```python
from build123d import *

# Parameters (mm, degrees)
SKETCH1_W               = 10
SKETCH1_H               = 10
BASE_FLANGE1_DEPTH      = 1
EDGE_FLANGE2_DEPTH      = 10
EDGE_FLANGE2_BEND_DEPTH = 10
EDGE_FLANGE3_DEPTH      = 10
EDGE_FLANGE3_BEND_DEPTH = 10
CUT_EXTRUDE1_DEPTH      = 10
SKETCH25_R              = 2.5
CUT_EXTRUDE2_DEPTH      = 10
SKETCH26_R              = 2.5
CUT_EXTRUDE3_DEPTH      = 10
SKETCH27_R              = 2.5
CUT_EXTRUDE4_DEPTH      = 1


# Sheet-metal steps are written as plain solids
with BuildPart() as part:
    # Sketch1 → Base-Flange1 (new body)
    with BuildSketch(Plane(origin=(0, 0, 0), x_dir=(1, 0, 0), z_dir=(0, 1, 0))):
        with Locations((0, 0.042787107)):
            Rectangle(SKETCH1_W, SKETCH1_H)
    extrude(amount=-BASE_FLANGE1_DEPTH)

    # Edge-Flange2 section (across the edge) → Edge-Flange2 (add)
    with BuildSketch(Plane(origin=(5.7366, -1, -5.042787107), x_dir=(-1, 0, 0), z_dir=(0, 0, 1))):
        with BuildLine():
            Line((-1, 0.7366), (-1, 9))
            Line((-1, 9), (0, 9))
            Line((0, 9), (0, 0.7366))
            ThreePointArc((0, 0.7366), (0.215745145, 0.215745145), (0.7366, 0))
            Line((0.7366, 0), (0.7366, -1))
            ThreePointArc((0.7366, -1), (-0.491361636, -0.491361636), (-1, 0.7366))
        make_face()
    extrude(amount=EDGE_FLANGE2_DEPTH)

    # Edge-Flange2 section 2 (across the edge) → Edge-Flange2 bend (add)
    with BuildSketch(Plane(origin=(-5.7366, -1, 4.957212893), x_dir=(1, 0, 0), z_dir=(0, 0, -1))):
        with BuildLine():
            Line((-1, 0.7366), (-1, 9))
            Line((-1, 9), (0, 9))
            Line((0, 9), (0, 0.7366))
            ThreePointArc((0, 0.7366), (0.215745145, 0.215745145), (0.7366, 0))
            Line((0.7366, 0), (0.7366, -1))
            ThreePointArc((0.7366, -1), (-0.491361636, -0.491361636), (-1, 0.7366))
        make_face()
    extrude(amount=EDGE_FLANGE2_BEND_DEPTH)

    # Edge-Flange3 section (across the edge) → Edge-Flange3 (add)
    with BuildSketch(Plane(origin=(6.7366, -10.7366, 4.957212893), x_dir=(0, 1, 0), z_dir=(0, 0, -1))):
        with BuildLine():
            Line((-1, 0.7366), (-1, 9))
            Line((-1, 9), (0, 9))
            Line((0, 9), (0, 0.7366))
            ThreePointArc((0, 0.7366), (0.215745145, 0.215745145), (0.7366, 0))
            Line((0.7366, 0), (0.7366, -1))
            ThreePointArc((0.7366, -1), (-0.491361636, -0.491361636), (-1, 0.7366))
        make_face()
    extrude(amount=EDGE_FLANGE3_DEPTH)

    # Edge-Flange3 section 2 (across the edge) → Edge-Flange3 bend (add)
    with BuildSketch(Plane(origin=(-6.7366, -10.7366, -5.042787107), x_dir=(0, 1, 0), z_dir=(0, 0, 1))):
        with BuildLine():
            Line((-1, 0.7366), (-1, 9))
            Line((-1, 9), (0, 9))
            Line((0, 9), (0, 0.7366))
            ThreePointArc((0, 0.7366), (0.215745145, 0.215745145), (0.7366, 0))
            Line((0.7366, 0), (0.7366, -1))
            ThreePointArc((0.7366, -1), (-0.491361636, -0.491361636), (-1, 0.7366))
        make_face()
    extrude(amount=EDGE_FLANGE3_BEND_DEPTH)

    # Sketch24 → Cut-Extrude1 (cut)
    with BuildSketch(Plane(origin=(0, -10.7366, 0), x_dir=(1, 0, 0), z_dir=(0, 1, 0))):
        with BuildLine():
            Line((15.7366, -4.957212893), (15.7366, 0.042787107))
            ThreePointArc((15.7366, 0.042787107), (14.57002385, -3.200318846), (11.6049, -4.957212893))
            Line((11.6049, -4.957212893), (15.7366, -4.957212893))
        make_face()
        with BuildLine():
            Line((15.7366, 5.042787107), (11.6049, 5.042787107))
            ThreePointArc((11.6049, 5.042787107), (14.57002385, 3.28589306), (15.7366, 0.042787107))
            Line((15.7366, 0.042787107), (15.7366, 5.042787107))
        make_face()
    cut_extrude1 = extrude(amount=-CUT_EXTRUDE1_DEPTH, mode=Mode.SUBTRACT)

    # Mirror1: Cut-Extrude1 across plane
    add(cut_extrude1.mirror(Plane(origin=(0, 0, 0), x_dir=(0, 0, 1), z_dir=(1, 0, 0))), mode=Mode.SUBTRACT)

    # Sketch25 → Cut-Extrude2 (cut)
    with BuildSketch(Plane(origin=(0, 0, 0), x_dir=(1, 0, 0), z_dir=(0, 1, 0))):
        with Locations(Location((0, 0, 0), (0, 0, 270))):
            Circle(SKETCH25_R)
    extrude(amount=-CUT_EXTRUDE2_DEPTH, mode=Mode.SUBTRACT)

    # Sketch26 → Cut-Extrude3 (cut)
    with BuildSketch(Plane(origin=(0, -10.7366, 0), x_dir=(1, 0, 0), z_dir=(0, 1, 0))):
        with Locations(Location((10.645360935, 0.042787107, 0), (0, 0, 270))):
            Circle(SKETCH26_R)
        with Locations(Location((-10.645360935, 0.042787107, 0), (0, 0, 270))):
            Circle(SKETCH26_R)
    extrude(amount=-CUT_EXTRUDE3_DEPTH, mode=Mode.SUBTRACT)

    # Sketch27 → Cut-Extrude4 (cut)
    with BuildSketch(Plane(origin=(6.7366, 0, 0), x_dir=(0, 0, -1), z_dir=(1, 0, 0))):
        with Locations(Location((0, -5.8683, 0), (0, 0, 90))):
            Circle(SKETCH27_R)
    cut_extrude4 = extrude(amount=-CUT_EXTRUDE4_DEPTH, mode=Mode.SUBTRACT)

    # Mirror2: Cut-Extrude4 across plane
    add(cut_extrude4.mirror(Plane(origin=(0, 0, 0), x_dir=(0, 0, 1), z_dir=(1, 0, 0))), mode=Mode.SUBTRACT)


solid = part.part
```
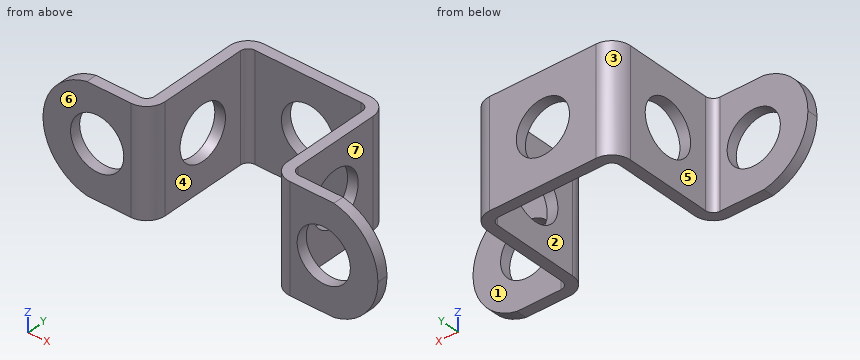
The model under review builds one solid part; all positions refer to its coordinate system, in mm. Face numbers are marked on the shaded views. A direction names the side the tool comes from. Coordinates: 2 decimals unless noted, no trailing zeros. Write each loop counter-clockwise with the first axis right and the second up, starting at its lowest first coordinate (ties: lowest second). Pieces come first, ordered by that corner, then holes. Notation, with made-up numbers: (31.5, -1.5) -> (79.5, -1.5) arc R25 cw to (79.5, 32.5) -> close; hole circle Ø2 at (1, -9). An arc over 180 degrees is marked (long way). One line per item, written item: value. Start each with the question number.
Q1. Add section C-C, the plane y = -7.75. Give the boundary of the cut face in (x, z).
Q2. Add section B-B, the plane x = 0. Give the boundary of the cut face in (y, z).
Q3. The part is to be moulded in two halves that separate along X. For the marked faces 1, 2 and 3, say which applies: +X half, -X half, draft (parallel to the pull), parting line (faces both ways), or undercut.
Q4. For the marked faces 4, 5, 6 and 7, list the 3-axis set-ups (+Z, -Z, +X, -X, +Y, -Y) from which the entire face can be reached by the end or side of a thin tool; tool diameter is ignored.
Q5. Add section A-A, the plane y = -9.5. Give the boundary of the cut face in (x, z).
Q6. Clearance check with flat-ended pins moving along their axes: P1, Ø5, axis at y = -5, z = -2.5, coming from the +X side; P2, Ø6, axis at y = -9.5, z = 3, coming from the +X side; P3, Ø4, axis at x = 10.5, z = 0.5, coming from the +Y side; P4, Ø4.5, axis at x = -10.65, z = -0.04, coming from the -Y side. State where each tip first meets the part, or that it passes through.
Q7. Add section D-D, the plane z = -2. Count the separate pieces of the cut face and the enclosed holes in it, then the cut area to 3 significant figures.
Q8. To check wall thickness, follow probe 1 along X at (y, z) = (-10, 3); probe 2 along X at (y, z) = (-11, 1.25); probe 3 along Y at (x, z) = (2, -1.75). State the ranges of each line that lie inside material, in increasing order.
Response:
1. outline: (-6.74, -5.04) -> (-5.74, -5.04) -> (-5.74, -1.65) -> (-6.74, -1.65) -> close; (-6.74, 1.65) -> (-5.74, 1.65) -> (-5.74, 4.96) -> (-6.74, 4.96) -> close; (5.74, -5.04) -> (6.74, -5.04) -> (6.74, -1.65) -> (5.74, -1.65) -> close; (5.74, 1.65) -> (6.74, 1.65) -> (6.74, 4.96) -> (5.74, 4.96) -> close
2. outline: (-1, -5.04) -> (0, -5.04) -> (0, -2.5) -> (-1, -2.5) -> close; (-1, 2.5) -> (0, 2.5) -> (0, 4.96) -> (-1, 4.96) -> close
3. face 1: draft
3. face 2: undercut
3. face 3: -X half
4. face 4: +Z, -Z, -Y
4. face 5: +Z, -Z, -X, +Y
4. face 6: +Z, -Z, +X, -X, -Y
4. face 7: +Z, -Z, +X, +Y
5. outline: (-6.74, -5.04) -> (-5.74, -5.04) -> (-5.74, 4.96) -> (-6.74, 4.96) -> close; (5.74, -5.04) -> (6.74, -5.04) -> (6.74, 4.96) -> (5.74, 4.96) -> close
6. P1: x = 6.74
6. P2: x = 15.73
6. P3: y = -10.74
6. P4: through
7. separate pieces: 6
7. enclosed holes: 0
7. area: 34.8 mm²
8. probe 1: -6.74 to -5.74, 5.74 to 6.74
8. probe 2: -15.57 to -12.79, -8.51 to -6.05, 6.05 to 8.51, 12.79 to 15.57
8. probe 3: -1 to 0
